Here's the drawing with two shaded views (mm, measured from the low corner). I have some questions. A direction names the side the tool comes from. Give positions to 0.01 mm unless a question says otherwise; leave off trailing zeros. Write each loop counter-clockwise with the first axis right and the second up, starting at its lowest first coordinate (ties: lowest second). Pieces come first, ordered by that corner, then holes.
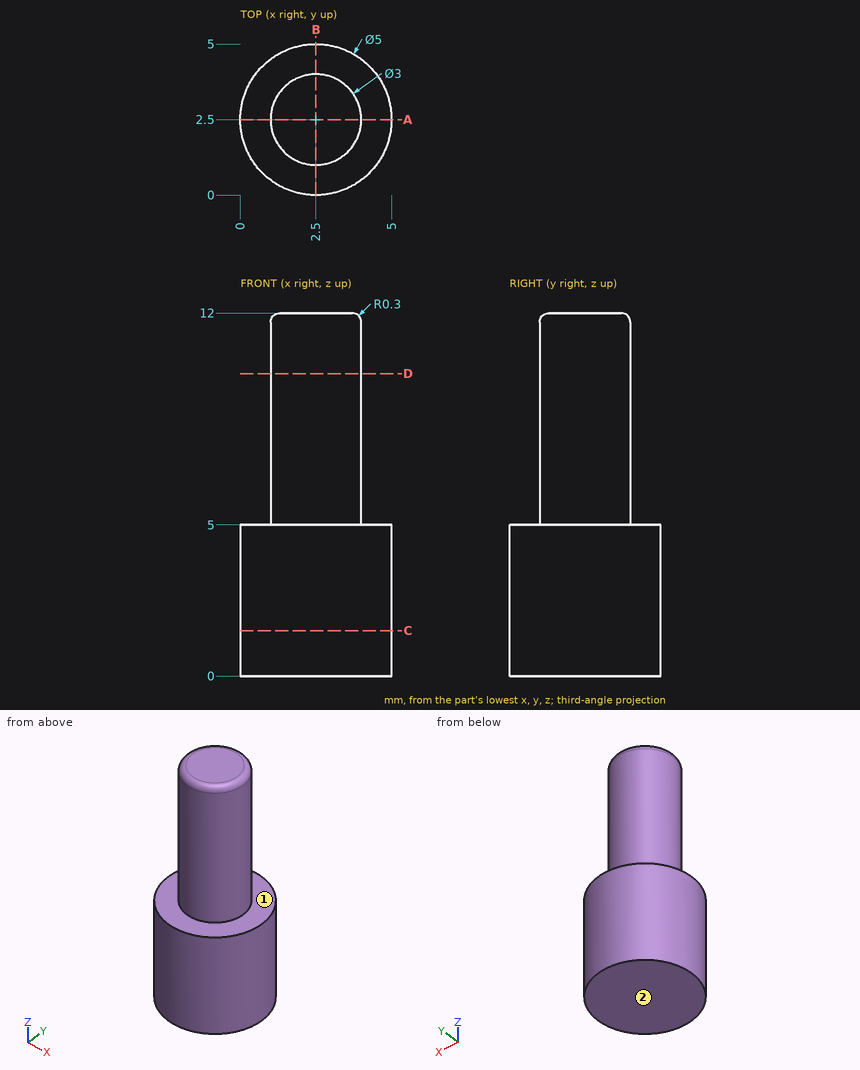
(1) Will these pins go through, and if not, where does the flat tip stop? P1, Ø3, axis at y = 4.5, z = 9.5, coming from the -X side; P2, Ø2, axis at y = 3.5, z = 4, coming from the -X side; P3, Ø2, axis at x = 1, z = 7, coming from the +Y side.
Returned:
P1: stops at x = 1.09
P2: stops at x = 0
P3: stops at y = 3.91
(2) If I drill on L1, parallel to Z at x = 3.15, y = 4.6; L2, parallel to Y at x = 1.8, z = 4; L3, parallel to Y at x = 3.05, z = 6.25, over which ranges is the centre line in solid material (lowest first)?
Returned:
L1: z = 0 to 5
L2: y = 0.1 to 4.9
L3: y = 1.1 to 3.9
(3) For the marked faces 1 and 2, which set-ups out of +Z, -Z, +X, -X, +Y, -Y let a thin tool reach every point of the face, with its end or its side?
Returned:
face 1: +Z
face 2: -Z, +X, -X, +Y, -Y
(4) Imagine slicing it at A-A, the plane y = 2.5. Write out the boundary of the cut face in (x, z).
Returned:
outline: (0, 0) - (5, 0) - (5, 5) - (4, 5) - (4, 11.7) arc R0.3 ccw to (3.7, 12) - (1.3, 12) arc R0.3 ccw to (1, 11.7) - (1, 5) - (0, 5) - close
(5) Imagine slicing it at D-D, the plane z = 10. Write out the boundary of the cut face in (x, y), plus the area to 3 significant figures.
Returned:
outline: circle Ø3 at (2.5, 2.5)
area: 7.07 mm2
(6) Imagine slicing it at C-C, the plane z = 1.5. Write out the boundary of the cut face in (x, y), plus the area to 3 significant figures.
Returned:
outline: circle Ø5 at (2.5, 2.5)
area: 19.6 mm2
